For this review, take the finished solid that the model builds, in its own axes (mm). A direction names the side the tool comes from. Give positions to 0.01 mm unless a question says otherwise; leave off trailing zeros. Order: outer loops, then holes, each group sorted by start corner. A loop starts at its lowest first (then second) coordinate and runs counter-clockwise, first axis right, second up. Notation, with made-up numbers: (-20.5, 75.25) - (16.5, 75.25) arc R14 cw to (16.5, 82.25) - close; hole circle Ø9 at (-15, -35). An arc over 180 degrees is marked (long way). Answer as a JSON object with one key per item and string values. Group by question number.
from build123d import *

# Parameters (mm, degrees)
F0_W     = 50
F0_H     = 10
F1_DEPTH = 5
F3_D     = 5.5
F4_W     = 3
F4_H     = 10
F5_DEPTH = 20
F7_D     = 5.5


with BuildPart() as f1:
    # F0 (on Top) → F1 (new body)
    with BuildSketch(Plane.XY):
        Rectangle(F0_W, F0_H)
    extrude(amount=F1_DEPTH)

    # F3 (through all)
    with Locations(Plane.XY.offset(5)):
        with Locations((-20, 0), (20, 0)):
            Hole(F3_D / 2)

    # F4 (on face) → F5 (join)
    with BuildSketch(Plane.XY.offset(5)):
        with Locations((-4.125, 0)):
            Rectangle(F4_W, F4_H)
        with Locations((4.125, 0)):
            Rectangle(F4_W, F4_H)
    extrude(amount=F5_DEPTH)

    # F7 (through all)
    with Locations(Plane(origin=(-5.625, 0, 0), x_dir=(0, -1, 0), z_dir=(-1, 0, 0))):
        with Locations((0, 20)):
            Hole(F7_D / 2)


solid = f1.part
1) For line 1 (X direction, y = 1.75, z = 1.5); line 2 (X direction, y = 1.5, z = 1.75); line 3 (X direction, y = -2.5, z = 18.5) (3 decimals), list the stretches that pass through material, from the lowest coordinate up.
2) Consider section B-B (x = 20). Give the boundary of the cut face in (y, z), plus the area to 3 significant figures.
3) Consider section A-A (z = 20). Give the boundary of the cut face in (x, y) (3 decimals), plus the area to 3 significant figures.
4) Consider section C-C (y = 0). Give the boundary of the cut face in (x, z) (3 decimals).
5) For faces 4 (the face through (0, 0, 5)), 5 (the face through (4.146, -0.358, 22.727)), 6 (the face through (-4, 0, 25)), 7 (the face through (15, 0, 5)), 8 (the face through (-5.625, 0, 15)), list the 3-axis set-ups (+Z, -Z, +X, -X, +Y, -Y) from which the entire face can be reached by the end or side of a thin tool; tool diameter is ignored.
6) For pin 1 (5 mm diameter, centred on x = -16.5, y = -3, fed in from -Z); pin 2 (3 mm diameter, centred on y = 4, z = 17.5, fed in from -X) (3 decimals); pin 3 (5 mm diameter, centred on x = 11, y = 1, fed in from +Z), all flat-tipped, find the tip position at first contact; note any pin that passes through.
7) Mouldability with a two-part tool opening along Y and no side actions: class faces 1 (the face through (22.747, 0.121, 2.465)), 2 (the face through (-2.625, 0, 15)), 3 (the face through (0, -5, 4)) as released by +Y, released by -Y, zero draft, split by the parting line, or undercut.
8) Consider section D-D (z = 10.5). Give the boundary of the cut face in (x, y) (3 decimals), plus the area to 3 significant figures.
Result set:
{
 "1": {"line 1": "x = -25 to -22.12, -17.88 to 17.88, 22.12 to 25", "line 2": "x = -25 to -22.3, -17.7 to 17.7, 22.3 to 25", "line 3": "x = -5.625 to -2.625, 2.625 to 5.625"},
 "2": {"outline": "(-5, 0) - (-2.75, 0) - (-2.75, 5) - (-5, 5) - close; (2.75, 0) - (5, 0) - (5, 5) - (2.75, 5) - close", "area": "22.5 mm2"},
 "3": {"outline": "(-5.625, -5) - (-2.625, -5) - (-2.625, -2.75) - (-5.625, -2.75) - close; (-5.625, 2.75) - (-2.625, 2.75) - (-2.625, 5) - (-5.625, 5) - close; (2.625, -5) - (5.625, -5) - (5.625, -2.75) - (2.625, -2.75) - close; (2.625, 2.75) - (5.625, 2.75) - (5.625, 5) - (2.625, 5) - close", "area": "27.0 mm2"},
 "4": {"outline": "(-25, 0) - (-22.75, 0) - (-22.75, 5) - (-25, 5) - close; (-17.25, 0) - (17.25, 0) - (17.25, 5) - (5.625, 5) - (5.625, 17.25) - (2.625, 17.25) - (2.625, 5) - (-2.625, 5) - (-2.625, 17.25) - (-5.625, 17.25) - (-5.625, 5) - (-17.25, 5) - close; (-5.625, 22.75) - (-2.625, 22.75) - (-2.625, 25) - (-5.625, 25) - close; (2.625, 22.75) - (5.625, 22.75) - (5.625, 25) - (2.625, 25) - close; (22.75, 0) - (25, 0) - (25, 5) - (22.75, 5) - close"},
 "5": {"face 4": "+Z, +Y, -Y", "face 5": "+X, -X", "face 6": "+Z, +X, -X, +Y, -Y", "face 7": "+Z, +X, +Y, -Y", "face 8": "+Z, -X, +Y, -Y"},
 "6": {"pin 1": "stops at z = 0", "pin 2": "stops at x = -5.625", "pin 3": "stops at z = 5"},
 "7": {"face 1": "undercut", "face 2": "zero draft", "face 3": "released by -Y"},
 "8": {"outline": "(-5.625, -5) - (-2.625, -5) - (-2.625, 5) - (-5.625, 5) - close; (2.625, -5) - (5.625, -5) - (5.625, 5) - (2.625, 5) - close", "area": "60.0 mm2"}
}
